from build123d import *

# Parameters (mm, degrees)
F1_DEPTH = 16
F2_R     = 3
F3_R     = 7.99999
F4_R     = 3
F4_W     = 13.7
F4_H     = 6.3
F5_DEPTH = 10


# Not quite as in the source:
# - a fillet or chamfer is up to 0.001 mm smaller than in the source, because OpenCascade refuses the exact size


with BuildPart() as f1:
    # F0 (on Front) → F1 (new body)
    with BuildSketch(Plane.XZ):
        with BuildLine():
            ThreePointArc((-25.7, 9.65), (-24.3502481093, 7.4100162997), (-24.4315048785, 4.7960624973))
            ThreePointArc((-24.4315048785, 4.7960624973), (-22.2846704688, -9.0000816848), (-9.85, -15.35))
            Line((-9.85, -15.35), (9.85, -15.35))
            ThreePointArc((9.85, -15.35), (20.7040890912, -10.8540890912), (25.2, 0))
            ThreePointArc((25.2, 0), (29.210075991, 8.7034493587), (38.4314464174, 11.3105680079))
            Line((38.4314464174, 11.3105680079), (45.8, 10.15))
            Line((45.8, 10.15), (45.8, 17.15))
            Line((45.8, 17.15), (-19.7, 17.15))
            Line((-19.7, 17.15), (-22.2, 19.85))
            Line((-22.2, 19.85), (-30.2, 19.85))
            Line((-30.2, 19.85), (-30.2, 15.15))
            Line((-30.2, 15.15), (-28.8, 15.15))
            Line((-28.8, 15.15), (-27.5, 16.65))
            Line((-27.5, 16.65), (-25.7, 16.65))
            Line((-25.7, 16.65), (-25.7, 9.65))
        make_face()
        with BuildLine():
            ThreePointArc((-9.85, -13.15), (-23, 0), (-9.85, 13.15))
            Line((-9.85, 13.15), (9.85, 13.15))
            ThreePointArc((9.85, 13.15), (23, 0), (9.85, -13.15))
            Line((9.85, -13.15), (-9.85, -13.15))
        make_face(mode=Mode.SUBTRACT)
    extrude(amount=F1_DEPTH)

    # F2
    f2_edges = [f1.edges().sort_by_distance(p)[0] for p in [
        (-30.2, -8, 19.85),
        (-22.2, -8, 19.85),
        (-19.7, -8, 17.15),
    ]]
    fillet(f2_edges, radius=F2_R)

    # F3 (radius 8 in the source; OpenCascade refuses exactly that, so slightly less here)
    f3_edges = [f1.edges().sort_by_distance(p)[0] for p in [
        (45.8, -16, 13.65),
        (45.8, 0, 13.65),
    ]]
    fillet(f3_edges, radius=F3_R)

    # F4 (on face) → F5 (cut)
    with BuildSketch(Plane.XY.offset(17.15)):
        with Locations((37.8, -8)):
            Circle(F4_R)
        with Locations((2.95, -8)):
            Rectangle(F4_W, F4_H)
    extrude(amount=-F5_DEPTH, mode=Mode.SUBTRACT)


solid = f1.part
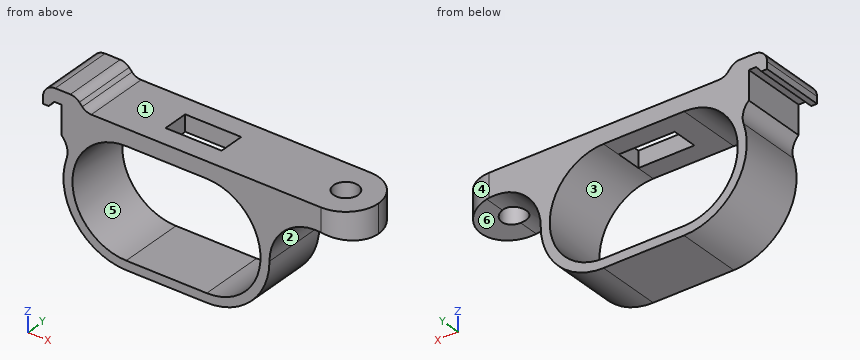
The model under review builds one solid part; all positions refer to its coordinate system, in mm. Face numbers are marked on the shaded views. A direction names the side the tool comes from. Round coordinates to 2 decimals unless told otherwise and drop trailing zeros. Loops run counter-clockwise (first coordinate to the right, second up) from the corner with the lowest first, then second, coordinate; pieces in that order, holes last. Notation, with made-up numbers: M 28,2.25 L 37,2.25 A27 cw 37,20.25 Z; hole C -12,-0.5 d9. An arc over 180 degrees is marked long. Answer as CSV lines item,"result".
1. We need section B-B (z = 8.5). Give the boundary of the cut face in (x, y).
Outcome:
outline,"M -24.79,-16 L -19.88,-16 L -19.88,0 L -24.79,0 Z; M 19.88,-16 L 28.98,-16 L 28.98,0 L 19.88,0 Z"
2. For the marked faces 4, 5 and 6, list the 3-axis set-ups (+Z, -Z, +X, -X, +Y, -Y) from which the entire face can be reached by the end or side of a thin tool; tool diameter is ignored.
Outcome:
face 4,"+Z, -Z, +X, +Y"
face 5,"+Y, -Y"
face 6,"-Z, +Y, -Y"
3. Draft analysis for pull direction Z (two halves, no side actions). For the marked faces 1, 2 and 3, state which applies: pulls with the +Z half, pulls with the -Z half, needs draft (parallel to the pull), parting line crosses it, or undercut.
Outcome:
face 1,"pulls with the +Z half"
face 2,"pulls with the -Z half"
face 3,"undercut"
4. We need section D-D (y = -1). Give the boundary of the cut face in (x, z), plus the area to 3 significant figures.
Outcome:
outline,"M -30.2,15.15 L -28.8,15.15 L -27.5,16.65 L -25.7,16.65 L -25.7,9.65 A4.62 cw -24.43,4.8 A15.35 ccw -9.85,-15.35 L 9.85,-15.35 A15.35 ccw 25.2,0 A11.45 cw 38.43,11.31 L 41.67,10.8 L 41.67,17.15 L -18.39,17.15 A3 cw -20.59,18.11 L -21.31,18.89 A3 ccw -23.51,19.85 L -27.2,19.85 A3 ccw -30.2,16.85 Z; hole M -9.85,-13.15 L 9.85,-13.15 A13.15 ccw 9.85,13.15 L -9.85,13.15 A13.15 ccw Z"
area,"627 mm2"
5. To check wall thickness, follow L1, parallel to X at y = -8, z = 14.25; L2, parallel to Y at x = 37.8, z = 13.5; L3, parallel to Z at x = 4, y = -12.5. State the ranges of each line that lie inside material, in increasing order. Write a range as [from, to].
Outcome:
L1,"x = [-25.7, -3.9], [9.8, 34.8], [40.8, 45.8]"
L2,"y = [-16, -11], [-5, 0]"
L3,"z = [-15.35, -13.15], [13.15, 17.15]"
6. We need section A-A (x = 9). Give the boundary of the cut face in (y, z), plus the area to 3 significant figures.
Outcome:
outline,"M -16,-15.35 L 0,-15.35 L 0,-13.15 L -16,-13.15 Z; M -16,13.15 L -11.15,13.15 L -11.15,17.15 L -16,17.15 Z; M -4.85,13.15 L 0,13.15 L 0,17.15 L -4.85,17.15 Z"
area,"74.0 mm2"
7. Insertion check: pin 1 Ø1.2 at (y, z) = (-6.5, 15) entering from -X; pin 2 Ø0.7 at (x, y) = (-30, -10) entering from -Z; pin 3 Ø5 at (x, y) = (-4.5, -10.5) entering from +Z; pin 4 Ø4 at (x, y) = (23, -14.5) entering from -Z. Each pin has a flat end and moves straight along its axis. Give the tip position at first contact, or say it passes through.
Outcome:
pin 1,"stops at x = -30.2"
pin 2,"stops at z = 15.15"
pin 3,"stops at z = 17.15"
pin 4,"stops at z = -10.55"
